Job drawing, mm, ordinate dimensions from the low corner. One solid piece. A direction names the side the tool comes from. Round coordinates to 2 decimals unless told otherwise and drop trailing zeros. Loops run counter-clockwise (first coordinate to the right, second up) from the corner with the lowest first, then second, coordinate; pieces in that order, holes last. Notation, with made-up numbers: M 40,-2.5 L 98,-2.5 A23 cw 98,10.5 Z; hole C 48.5,-9 d8. An arc over 180 degrees is marked long. Use one line per item in the form item = value. Start each with the question number.
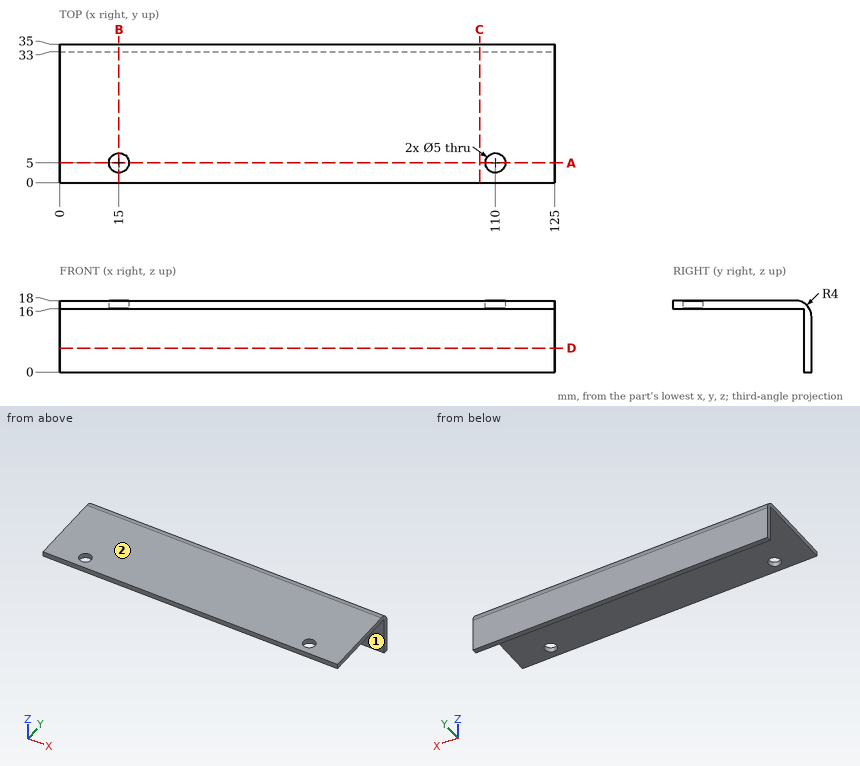
Q1. Saw through at C-C (x = 106). Give the cut face in (y, z).
Q2. Saw through at D-D (z = 6). Give the cut face in (x, y).
Q3. Saw through at B-B (x = 15). Give the cut face in (y, z), and give its area (3 significant figures).
Q4. Drop flat-ended pins along their axis: P1, Ø10, axis at x = 64, y = 25, coming from the -Z side; P2, Ø5, axis at x = 26, z = 5, coming from the -Y side. Give the stop position or say it passes through.
Q5. Tool access for the marked faces 1 and 2: list every direction of +Z, -Z, +X, -X, +Y, -Y with a clear straight run to the whole face (end or side of a thin tool).
Q6. Wall check: probe 1 along Z at (x, y) = (114, 10); probe 2 along Y at (x, z) = (110, 17.65); probe 3 along Y at (x, z) = (107, 1). Give the ranges that are in metal, low to high.
Q7. Saw through at A-A (y = 5). Give the cut face in (x, z).
Filled in:
q1.outline = M 0,16 L 33,16 L 33,0 L 35,0 L 35,14 A4 ccw 31,18 L 0,18 Z
q2.outline = M 0,33 L 125,33 L 125,35 L 0,35 Z
q3.outline = M 0,16 L 2.5,16 L 2.5,18 L 0,18 Z; M 7.5,16 L 33,16 L 33,0 L 35,0 L 35,14 A4 ccw 31,18 L 7.5,18 Z
q3.area = 88.6 mm²
q4.P1 = 16
q4.P2 = 33
q5.face_1 = -Z, +X, -X, -Y
q5.face_2 = +Z, +X, -X, +Y, -Y
q6.probe_1 = 16 to 18
q6.probe_2 = 0 to 2.5, 7.5 to 32.64
q6.probe_3 = 33 to 35
q7.outline = M 0,16 L 12.5,16 L 12.5,18 L 0,18 Z; M 17.5,16 L 107.5,16 L 107.5,18 L 17.5,18 Z; M 112.5,16 L 125,16 L 125,18 L 112.5,18 Z
